```python
from build123d import *

# Parameters (mm, degrees)
SKETCH3_W           = 155
SKETCH3_H           = 30
BOSS_EXTRUDE3_DEPTH = 10
SKETCH4_W           = 10
SKETCH4_H           = 10
BOSS_EXTRUDE4_DEPTH = 25
SKETCH6_R           = 2
CUT_EXTRUDE1_DEPTH  = 10
SKETCH7_R           = 1.5
SKETCH7_R_2         = 1.85
CUT_EXTRUDE2_DEPTH  = 10


with BuildPart() as part:
    # Sketch3 → Boss-Extrude3 (new body)
    with BuildSketch(Plane(origin=(0, 0, 0), x_dir=(1, 0, 0), z_dir=(0, 1, 0))):
        with Locations((23.197278912, 148.962585034)):
            Rectangle(SKETCH3_W, SKETCH3_H)
    extrude(amount=BOSS_EXTRUDE3_DEPTH)

    # Sketch4 → Boss-Extrude4 (add)
    with BuildSketch(Plane(origin=(0, 10, 0), x_dir=(1, 0, 0), z_dir=(0, 1, 0))):
        with Locations((-49.302721088, 158.962585034)):
            Rectangle(SKETCH4_W, SKETCH4_H)
        with Locations((-49.302721088, 138.962585034)):
            Rectangle(SKETCH4_W, SKETCH4_H)
        with Locations((95.697278912, 158.962585034)):
            Rectangle(SKETCH4_W, SKETCH4_H)
        with Locations((95.697278912, 138.962585034)):
            Rectangle(SKETCH4_W, SKETCH4_H)
    extrude(amount=BOSS_EXTRUDE4_DEPTH)

    # Sketch6 → Cut-Extrude1 (cut)
    with BuildSketch(Plane(origin=(0, 35, 0), x_dir=(1, 0, 0), z_dir=(0, 1, 0))):
        with Locations((95.697278912, 138.962585034)):
            Circle(SKETCH6_R)
        with Locations((95.697278912, 158.962585034)):
            Circle(SKETCH6_R)
        with Locations((-49.302721088, 138.962585034)):
            Circle(SKETCH6_R)
        with Locations((-49.302721088, 158.962585034)):
            Circle(SKETCH6_R)
    extrude(amount=-CUT_EXTRUDE1_DEPTH, mode=Mode.SUBTRACT)

    # Sketch7 → Cut-Extrude2 (cut)
    with BuildSketch(Plane(origin=(0, 10, 0), x_dir=(1, 0, 0), z_dir=(0, 1, 0))):
        with Locations((95.697278912, 148.962585034)):
            Circle(SKETCH7_R)
        with Locations((82.297278912, 139.062585034)):
            Circle(SKETCH7_R_2)
        with Locations((82.297278912, 159.062585034)):
            Circle(SKETCH7_R_2)
        with Locations((-49.302721088, 148.962585034)):
            Circle(SKETCH7_R)
        with Locations((-9.202721088, 144.062585034)):
            Circle(SKETCH7_R_2)
    extrude(amount=-CUT_EXTRUDE2_DEPTH, mode=Mode.SUBTRACT)


solid = part.part
```
CAD build for the part. Positions are in the model's coordinates, mm. A direction names the side the tool comes from. Give positions to 0.01 mm unless a question says otherwise; leave off trailing zeros. Order: outer loops, then holes, each group sorted by start corner. A loop starts at its lowest first (then second) coordinate and runs counter-clockwise, first axis right, second up.
(1) Drill centre lines: L1, parallel to X at y = 31, z = -160.5; L2, parallel to X at y = 9.5, z = -150.25; L3, parallel to Z at x = -48, y = 12.5. Where is each one in solid material? Low to high.
(2) Saw through at A-A, the plane y = 12.5. Give the cut face in (x, z).
(3) Tool access for faces 4 (the flat face through (-44.303, 22, -159)), 5 (the flat face through (96, 22, -143.963)), 6 (the flat face through (-49, 25, -139)), 7 (the flat face through (-47, 35, -159)): list every direction of +Z, -Z, +X, -X, +Y, -Y with a clear straight run to the whole face (end or side of a thin tool).
(4) Saw through at B-B, the plane y = 28. Give the cut face in (x, z), then the cut area to 3 significant figures.
(5) Mould opens along X. For faces 1 (the flat face through (93, 35, -139)), 2 (the flat face through (-54.303, 9, -149)), 3 (the cylindrical face through (96.5, 5.07, -150.23)) say: released by +X, released by -X, zero draft, split by the parting line, or undercut.
(6) Saw through at C-C, the plane x = 0. Give the cut face in (y, z), then the cut area to 3 significant figures.
(7) Flat gauge pins, fed straight in: pin 1 (1.8 mm diameter, centred on x = 95.7, z = -148.96, fed in from -Y); pin 2 (2 mm diameter, centred on x = 95, z = -139, fed in from +Y); pin 3 (6 mm diameter, centred on x = 15.5, z = -156, fed in from +Y). Where does each tip first touch, or does it go through?
Results found:
1. L1: x = -54.3 to -50.58, -48.02 to -44.3, 90.7 to 94.42, 96.98 to 100.7
1. L2: x = -54.3 to -50.07, -48.53 to 94.93, 96.47 to 100.7
1. L3: z = -163.96 to -153.96, -143.96 to -133.96
2. outline: (-54.3, -163.96) - (-44.3, -163.96) - (-44.3, -153.96) - (-54.3, -153.96) - close; (-54.3, -143.96) - (-44.3, -143.96) - (-44.3, -133.96) - (-54.3, -133.96) - close; (90.7, -163.96) - (100.7, -163.96) - (100.7, -153.96) - (90.7, -153.96) - close; (90.7, -143.96) - (100.7, -143.96) - (100.7, -133.96) - (90.7, -133.96) - close
3. face 4: +Z, -Z, +Y
3. face 5: +X, -X, +Y
3. face 6: +Y
3. face 7: +Z, -Z, +X, -X, +Y
4. outline: (-54.3, -163.96) - (-44.3, -163.96) - (-44.3, -153.96) - (-54.3, -153.96) - close; (-54.3, -143.96) - (-44.3, -143.96) - (-44.3, -133.96) - (-54.3, -133.96) - close; (90.7, -163.96) - (100.7, -163.96) - (100.7, -153.96) - (90.7, -153.96) - close; (90.7, -143.96) - (100.7, -143.96) - (100.7, -133.96) - (90.7, -133.96) - close; hole circle Ø4 at (-49.3, -158.96); hole circle Ø4 at (-49.3, -138.96); hole circle Ø4 at (95.7, -158.96); hole circle Ø4 at (95.7, -138.96)
4. area: 350 mm2
5. face 1: zero draft
5. face 2: released by -X
5. face 3: undercut
6. outline: (0, -163.96) - (10, -163.96) - (10, -133.96) - (0, -133.96) - close
6. area: 300 mm2
7. pin 1: passes through
7. pin 2: stops at y = 25
7. pin 3: stops at y = 10
